Check sheet for the modelled part. Datum: model origin and axes. Units: mm. A direction names the side the tool comes from. Coordinates: 2 decimals unless noted, no trailing zeros. Loops run counter-clockwise (first coordinate to the right, second up) from the corner with the lowest first, then second, coordinate; pieces in that order, holes last. Notation, with made-up numbers: M -10.75,44.25 L 25.25,44.25 A13 cw 25.25,56.25 Z; hole C 80,-4.75 d1. An arc over 180 degrees is marked long. Answer in a Markdown table with one row per item. Add a question column.
```python
from build123d import *

# Parameters (mm, degrees)
SKETCH_1_R          = 1.3
EXTRUDE_1_DEPTH     = 3
SKETCH_2_R          = 1.6
CUT_EXTRUDE_1_DEPTH = 33.790082592


with BuildPart() as part:
    # 草图1 → 凸台-拉伸1 (new body)
    with BuildSketch(Plane(origin=(0, 0, 0), x_dir=(-1, 0, 0), z_dir=(0, 0, -1))):
        with BuildLine():
            Line((8.503321513, 25.001), (-5.486589193, 25.001))
            ThreePointArc((-5.486589193, 25.001), (-14.325423958, 21.339834765), (-17.986589193, 12.501))
            Line((-17.986589193, 12.501), (-17.986589193, 12.5))
            ThreePointArc((-17.986589193, 12.5), (-14.325423958, 3.661165235), (-5.486589193, 0))
            Line((-5.486589193, 0), (8.503321493, 0))
            ThreePointArc((8.503321493, 0), (17.342156257, 3.661165235), (21.003321493, 12.5))
            ThreePointArc((21.003321493, 12.5), (17.342509831, 21.339481206), (8.503321513, 25.001))
        make_face()
        with Locations(Location((1.487905971, 22.0005, 0), (0, 0, 180))):
            Circle(SKETCH_1_R, mode=Mode.SUBTRACT)
        with Locations(Location((1.487905971, 2.9995, 0), (0, 0, 180))):
            Circle(SKETCH_1_R, mode=Mode.SUBTRACT)
        Polygon((-11.997794717, 15), (-9.996894717, 15), (-9.996894717, 18.6), (13.002605283, 18.6), (13.002605283, 6.4), (-9.996894717, 6.4), (-9.996894717, 10.001), (-11.997794717, 10.001), align=None, mode=Mode.SUBTRACT)
    extrude(amount=-EXTRUDE_1_DEPTH)

    # 草图2 → 切除-拉伸1 (cut, through all)
    with BuildSketch(Plane.XY.offset(3)):
        with Locations((-1.487905971, 22.0005)):
            Circle(SKETCH_2_R)
        with Locations((-1.487905971, 2.9995)):
            Circle(SKETCH_2_R)
    extrude(amount=-CUT_EXTRUDE_1_DEPTH, mode=Mode.SUBTRACT)


solid = part.part
```
Q1. Access from +Z, -Z, +X, -X, +Y, -Y to the whole of each face (thin tool, end or side, straight path). Record for faces 1 (the face through (-2, 6.4, 1)), 2 (the face through (-6, 21, 3)).
Q2. Thickness scan on L1, parallel to Y at x = -4, z = 1.6; L2, parallel to Y at x = -10, z = 2.2; L3, parallel to X at y = 7, z = 2. Record the ranges inside material, lowest first.
Q3. Cross-section at B-B (x = -0.5). Record the cut outline in (y, z).
Q4. Cross-section at A-A (y = 21.5). Record the cut outline in (x, z).
Q5. Cross-section at D-D (x = 8.5). Record the cut outline in (y, z).
Q6. Cross-section at C-C (z = 1). Count the separate pieces of the cut face and the enclosed holes in it, plus the area to 3 significant figures.
Q7. Go/stop test with flat-tipped pins: pin 1 (1.9 mm diameter, centred on x = -1.49, y = 22, fed in from -Z); pin 2 (1 mm diameter, centred on x = -15, z = 1.5, fed in from -Y); pin 3 (0.9 mm diameter, centred on y = 9.5, z = 1, fed in from +X). Record where each tip stops, or that it passes through.
Answer key:
| question | item | result |
|---|---|---|
| 1 | face 1 | +Z, -Z |
| 1 | face 2 | +Z, +X, -X, +Y, -Y |
| 2 | L1 | 0 to 6.4, 18.6 to 25 |
| 2 | L2 | 0.09 to 6.4, 18.6 to 24.91 |
| 2 | L3 | -19.73 to -13, 10 to 16.71 |
| 3 | outline | M 0,0 L 1.74,0 L 1.74,3 L 0,3 Z; M 4.26,0 L 6.4,0 L 6.4,3 L 4.26,3 Z; M 18.6,0 L 20.74,0 L 20.74,3 L 18.6,3 Z; M 23.26,0 L 25,0 L 25,3 L 23.26,3 Z |
| 4 | outline | M -17.18,0 L -3.01,0 L -3.01,3 L -17.18,3 Z; M 0.03,0 L 14.16,0 L 14.16,3 L 0.03,3 Z |
| 5 | outline | M 0.37,0 L 6.4,0 L 6.4,3 L 0.37,3 Z; M 18.6,0 L 24.63,0 L 24.63,3 L 18.6,3 Z |
| 6 | separate pieces | 1 |
| 6 | enclosed holes | 3 |
| 6 | area | 534 mm^2 |
| 7 | pin 1 | through |
| 7 | pin 2 | y = 1.53 |
| 7 | pin 3 | x = 17.72 |
